Work out the finished part from the listing and answer in its coordinate system (mm). A direction names the side the tool comes from. Round coordinates to 2 decimals unless told otherwise and drop trailing zeros. Order: outer loops, then holes, each group sorted by start corner. A loop starts at its lowest first (then second) coordinate and runs counter-clockwise, first axis right, second up. Notation, with made-up numbers: M 17,2.25 L 25,2.25 A7 ccw 25,14.25 Z; hole C 61,20.5 d7. An arc over 180 degrees is marked long. Answer as a JSON object with one key per item and string values. Group by question number.
from build123d import *

# Parameters (mm, degrees)
SKETCH5_W            = 38.79143083
SKETCH5_H            = 48
CUT_EXTRUDE1_DEPTH   = 30
BOSS_EXTRUDE1_START  = -50
BOSS_EXTRUDE1_DEPTH  = 50
M5_CLEARANCE_HOLE1_D = 5.5


with BuildPart() as part:
    # Sketch1 → Revolve1 (revolve)
    with BuildSketch(Plane.XY, mode=Mode.PRIVATE) as revolve1_sk:
        Polygon((-24, 0), (-24, 50), (-16, 50), (-16, 34), (-13, 34), (-13, 30), (-16, 30), (-20, 30), (-20, 0), align=None)
    revolve(revolve1_sk.sketch.rotate(Axis((0, 0, 0), (0, 1, 0)), 270), axis=Axis((0, 0, 0), (0, 1, 0)))

    # Sketch5 → Cut-Extrude1 (cut)
    with BuildSketch(Plane(origin=(0, 0, 0), x_dir=(1, 0, 0), z_dir=(0, 1, 0))):
        with Locations((-19.395715415, 0)):
            Rectangle(SKETCH5_W, SKETCH5_H)
    extrude(amount=CUT_EXTRUDE1_DEPTH, mode=Mode.SUBTRACT)

    # Sketch6 → Boss-Extrude1 (add)
    with BuildSketch(Plane(origin=(0, 50, 0), x_dir=(1, 0, 0), z_dir=(0, 1, 0)).offset(BOSS_EXTRUDE1_START)):
        with BuildLine():
            Line((0, -24), (20.5, -24))
            ThreePointArc((20.5, -24), (27.571067812, -21.071067812), (30.5, -14))
            Line((30.5, -14), (30.5, 14))
            ThreePointArc((30.5, 14), (27.571067812, 21.071067812), (20.5, 24))
            Line((20.5, 24), (0, 24))
            ThreePointArc((0, 24), (24, 0), (0, -24))
        make_face()
    extrude(amount=BOSS_EXTRUDE1_DEPTH)

    # M5 Clearance Hole1 (through all)
    with Locations(Plane(origin=(0, 0, 0), x_dir=(-1, 0, 0), z_dir=(0, -1, 0))):
        with Locations((-22.5, -16), (-22.5, 16)):
            Hole(M5_CLEARANCE_HOLE1_D / 2)


solid = part.part
Item 1: A tool of negligible diameter and unlimited length cuts with its end or side. For faces 4 (the cylindrical face through (20, 15, 0)), 5 (the cylindrical face through (15.62, 41.89, 3.47)), 6 (the flat face through (0, 15, 22)), from which of +Z, -Z, +X, -X, +Y, -Y can it reach the whole face along a straight path? Write none if from no direction.
Item 2: Find section A-A (z = 0). Give the vertices of the cut face in (x, y), and give its area (3 significant figures).
Item 3: The mould has two halves that part along X. Classify faces 1 (the cylindrical face through (7.91, 31.972, 10.316)), 2 (the flat face through (10, 25, 24)), 3 (the cylindrical face through (-23.994, 40.14, -0.528)): +X half, -X half, draft (parallel to the pull), parting line (faces both ways), or undercut.
Item 4: Consider L1, parallel to Z at x = 22.5, y = 15; L2, parallel to X at y = 21.5, z = 17; L3, parallel to Y at x = -20.5, z = -2.5. Determine where each line is inside the solid, lowest interval first.
Item 5: Find section D-D (x = -3). Give the vertices of the cut face in (y, z), and give its area (3 significant figures).
Item 6: Find section B-B (y = 31.5). Give the vertices of the cut face in (x, z).
Item 7: Each of these flat-tipped pins is pushed along its axis until it touches: pin 1 (7 mm diameter, centred on x = 22.5, z = 16, fed in from +Y); pin 2 (1.2 mm diameter, centred on y = 10.5, z = -23, fed in from -X); pin 3 (13 mm diameter, centred on x = 0, z = 11.5, fed in from -Y); pin 4 (10 mm diameter, centred on x = -0.5, z = 7.5, fed in from -Y). Where does it stop, or does it pass through?
Item 8: Find section C-C (y = 26.5). Give the vertices of the cut face in (x, z), and give its area (3 significant figures).
Responses:
{
 "1": {"face 4": "-X, -Y", "face 5": "+Y", "face 6": "+Z, -Z, -X, -Y"},
 "2": {"outline": "M -24,30 L -13,30 L -13,34 L -16,34 L -16,50 L -24,50 Z; M 13,30 L 20,30 L 20,0 L 30.5,0 L 30.5,50 L 16,50 L 16,34 L 13,34 Z", "area": "789 mm^2"},
 "3": {"face 1": "undercut", "face 2": "draft", "face 3": "-X half"},
 "4": {"L1": "z = -23.8 to -18.75, -13.25 to 13.25, 18.75 to 23.8", "L2": "x = 10.54 to 19.94, 25.06 to 30.04", "L3": "y = 30 to 50"},
 "5": {"outline": "M 30,-23.81 L 50,-23.81 L 50,-15.72 L 34,-15.72 L 34,-12.65 L 30,-12.65 Z; M 30,12.65 L 34,12.65 L 34,15.72 L 50,15.72 L 50,23.81 L 30,23.81 Z", "area": "348 mm^2"},
 "6": {"outline": "M 0,-24 L 20.5,-24 A10 ccw 30.5,-14 L 30.5,14 A10 ccw 20.5,24 L 0,24 A24 ccw Z; hole C 0,0 d26; hole C 22.5,-16 d5.5; hole C 22.5,16 d5.5"},
 "7": {"pin 1": "stops at y = 50", "pin 2": "stops at x = 0", "pin 3": "stops at y = 30", "pin 4": "passes through"},
 "8": {"outline": "M 0,-24 L 20.5,-24 A10 ccw 30.5,-14 L 30.5,14 A10 ccw 20.5,24 L 0,24 L 0,20 A20 cw 0,-20 Z; hole C 22.5,-16 d5.5; hole C 22.5,16 d5.5", "area": "745 mm^2"}
}
